The listing builds one solid part. Answer for the finished solid, in the listing's coordinates (mm). A direction names the side the tool comes from. Give positions to 0.01 mm unless a question says otherwise; leave off trailing zeros. Order: outer loops, then holes, each group sorted by start corner. A loop starts at its lowest first (then second) coordinate and runs counter-clockwise, first axis right, second up. Notation, with made-up numbers: (-32, 75) - (26, 75) arc R22 cw to (26, 85) - close; hole circle Ø7 at (29.5, 15.5). An arc over 180 degrees is marked (long way). Answer in a Markdown table with one row per item.
from build123d import *

# Parameters (mm, degrees)
SKETCH1_R                            = 2.0193
BOSS_EXTRUDE1_DEPTH                  = 20.9931
F_10_32_TAPPED_HOLE1_D               = 4.0386
F_10_32_TAPPED_HOLE1_DEPTH           = 11.938
F_10_32_TAPPED_HOLE1_TIP             = 1.213317848
F_10_32_TAPPED_HOLE1_ON_FACE_2_D     = 4.0386
F_10_32_TAPPED_HOLE1_ON_FACE_2_DEPTH = 11.938
F_10_32_TAPPED_HOLE1_ON_FACE_2_TIP   = 1.213317848
SKETCH4_R                            = 8.89
SKETCH4_R_2                          = 6.35
CUT_EXTRUDE_THIN1_DEPTH              = 7.9375
SKETCH5_R                            = 7.665000037
SKETCH5_R_2                          = 5.125000037
CUT_EXTRUDE_THIN2_DEPTH              = 7.112


with BuildPart() as part:
    # Sketch1 → Boss-Extrude1 (new, symmetric)
    with BuildSketch(Plane.XY):
        with BuildLine():
            ThreePointArc((6.874999966, 0), (6.860422465, 0.447468582), (6.816751782, 0.893039571))
            Line((6.816751782, 0.893039571), (4.181770846, 5.456960429))
            ThreePointArc((4.181770846, 5.456960429), (3.437499983, 5.953924622), (2.634980936, 6.35))
            Line((2.634980936, 6.35), (-2.634980936, 6.35))
            ThreePointArc((-2.634980936, 6.35), (-3.437499983, 5.953924622), (-4.181770846, 5.456960429))
            Line((-4.181770846, 5.456960429), (-6.816751782, 0.893039571))
            ThreePointArc((-6.816751782, 0.893039571), (-6.874999966, 0), (-6.816751782, -0.893039571))
            Line((-6.816751782, -0.893039571), (-4.181770846, -5.456960429))
            ThreePointArc((-4.181770846, -5.456960429), (-3.437499983, -5.953924622), (-2.634980936, -6.35))
            Line((-2.634980936, -6.35), (2.634980936, -6.35))
            ThreePointArc((2.634980936, -6.35), (3.437499983, -5.953924622), (4.181770846, -5.456960429))
            Line((4.181770846, -5.456960429), (6.816751782, -0.893039571))
            ThreePointArc((6.816751782, -0.893039571), (6.860422465, -0.447468582), (6.874999966, 0))
        make_face()
        with Locations(Location((0, 0, 0), (0, 0, 180))):
            Circle(SKETCH1_R, mode=Mode.SUBTRACT)
    extrude(amount=BOSS_EXTRUDE1_DEPTH, both=True)

    # #10-32 Tapped Hole1
    with Locations(Plane.XY.offset(20.9931)):
        with Locations((0, 0)):
            Hole(F_10_32_TAPPED_HOLE1_D / 2, depth=F_10_32_TAPPED_HOLE1_DEPTH)
            with Locations((0, 0, -(F_10_32_TAPPED_HOLE1_DEPTH + F_10_32_TAPPED_HOLE1_TIP / 2))):  # 118° drill point
                Cone(0, F_10_32_TAPPED_HOLE1_D / 2, F_10_32_TAPPED_HOLE1_TIP, mode=Mode.SUBTRACT)

    # #10-32 Tapped Hole1 on face 2
    with Locations(Plane.XY.offset(-20.9931)):
        with Locations((0, 0)):
            Hole(F_10_32_TAPPED_HOLE1_ON_FACE_2_D / 2, depth=F_10_32_TAPPED_HOLE1_ON_FACE_2_DEPTH)
            with Locations((0, 0, -(F_10_32_TAPPED_HOLE1_ON_FACE_2_DEPTH + F_10_32_TAPPED_HOLE1_ON_FACE_2_TIP / 2))):  # 118° drill point
                Cone(0, F_10_32_TAPPED_HOLE1_ON_FACE_2_D / 2, F_10_32_TAPPED_HOLE1_ON_FACE_2_TIP, mode=Mode.SUBTRACT)

    # Sketch4 → Cut-Extrude-Thin1 (cut)
    with BuildSketch(Plane.XY.offset(20.9931)):
        Circle(SKETCH4_R)
        Circle(SKETCH4_R_2, mode=Mode.SUBTRACT)
    extrude(amount=-CUT_EXTRUDE_THIN1_DEPTH, mode=Mode.SUBTRACT)

    # Sketch5 → Cut-Extrude-Thin2 (cut)
    with BuildSketch(Plane(origin=(0, 0, -20.9931), x_dir=(-1, 0, 0), z_dir=(0, 0, -1))):
        Circle(SKETCH5_R)
        Circle(SKETCH5_R_2, mode=Mode.SUBTRACT)
    extrude(amount=-CUT_EXTRUDE_THIN2_DEPTH, mode=Mode.SUBTRACT)


solid = part.part
Item 1: Which of the six approach directions +Z, -Z, +X, -X, +Y, -Y give full straight-line access (tool end or side, diameter ignored) to faces 1 (the face through (3, -6, 13.056)), 2 (the face through (3, 6, 13.056)), 3 (the face through (-6.5, 0, 13.056)), 4 (the face through (-3, 6, 13.056))?
Answer block:
| item | result |
|---|---|
| face 1 | +Z, +X, -Y |
| face 2 | +Z, +X, +Y |
| face 3 | +Z, -X |
| face 4 | +Z, -X, +Y |
Item 2: Find section B-B on z = -5. Write down the section's boundary in (x, y) (3 decimals).
Answer block:
| item | result |
|---|---|
| outline | (-6.817, -0.893) - (-4.182, -5.457) arc R6.875 ccw to (-2.635, -6.35) - (2.635, -6.35) arc R6.875 ccw to (4.182, -5.457) - (6.817, -0.893) arc R6.875 ccw to (6.817, 0.893) - (4.182, 5.457) arc R6.875 ccw to (2.635, 6.35) - (-2.635, 6.35) arc R6.875 ccw to (-4.182, 5.457) - (-6.817, 0.893) arc R6.875 ccw to start; hole circle Ø4.039 at (0, 0) |
Item 3: Determine the mould class of faces 5 (the face through (-2, 2, 20.993)), 6 (the face through (-1.38, -6.2, 17.08)), 7 (the face through (-1.926, -0.607, -0.294)), 8 (the face through (-6.875, 0.013, -0.224)) for opening direction X: pulls with the +X half, pulls with the -X half, needs draft (parallel to the pull), parting line crosses it, or undercut.
Answer block:
| item | result |
|---|---|
| face 5 | needs draft |
| face 6 | parting line crosses it |
| face 7 | undercut |
| face 8 | pulls with the -X half |
Item 4: Consider line 1 (Y direction, x = 0, z = 10); line 2 (Z direction, x = -2.5, y = 5.5); line 3 (X direction, y = 1.25, z = -8). Determine where each line is inside the solid, lowest interval first.
Answer block:
| item | result |
|---|---|
| line 1 | -6.35 to -2.02, 2.02 to 6.35 |
| line 2 | -13.88 to 20.99 |
| line 3 | -6.61 to -1.59, 1.59 to 6.61 |
Item 5: Find section A-A on y = 0.5. Write down the section's boundary in (x, z), then the cut area to 3 significant figures.
Answer block:
| item | result |
|---|---|
| outline | (-6.86, -13.88) - (-5.1, -13.88) - (-5.1, -20.99) - (-1.96, -20.99) - (-1.96, 20.99) - (-6.33, 20.99) - (-6.33, 13.06) - (-6.86, 13.06) - close; (1.96, -20.99) - (5.1, -20.99) - (5.1, -13.88) - (6.86, -13.88) - (6.86, 13.06) - (6.33, 13.06) - (6.33, 20.99) - (1.96, 20.99) - close |
| area | 378 mm² |
Item 6: Find section D-D on y = 4. Write down the section's boundary in (x, z).
Answer block:
| item | result |
|---|---|
| outline | (-5.02, -13.88) - (-3.2, -13.88) - (-3.2, -20.99) - (3.2, -20.99) - (3.2, -13.88) - (5.02, -13.88) - (5.02, 13.06) - (4.93, 13.06) - (4.93, 20.99) - (-4.93, 20.99) - (-4.93, 13.06) - (-5.02, 13.06) - close |
Item 7: Each of these flat-tipped pins is pushed along its axis until it touches: P1, Ø8, axis at x = 5, z = -8.5, coming from the -Y side; P2, Ø5, axis at y = -5, z = 1.5, coming from the -X side. Where does it stop, or does it pass through?
Answer block:
| item | result |
|---|---|
| P1 | y = -6.35 |
| P2 | x = -5.89 |
